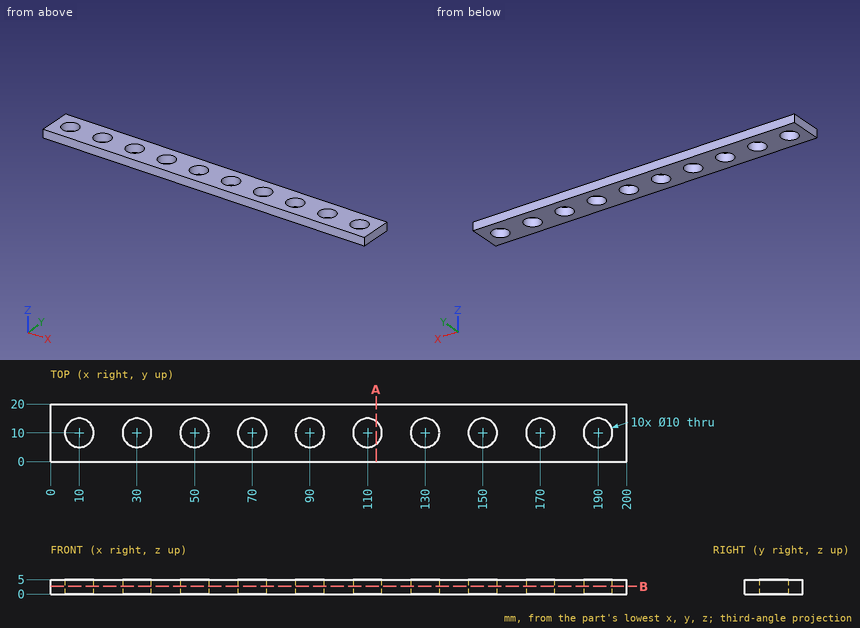
Geometry: see drawing. Coordinates: mm, zero at the bounding-box minimum. Round coordinates to 2 decimals unless told otherwise and drop trailing zeros. Write each loop counter-clockwise with the first axis right and the second up, starting at its lowest first coordinate (ties: lowest second). Pieces come first, ordered by that corner, then holes.
Item 1: Section query B-B (z = 2.65). Give the number of separate pieces and of enclosed holes in the cut face, plus the area to 3 significant figures.
Item 2: Material intervals for L1, parallel to Y at x = 190, z = 3.6; L2, parallel to Y at x = 148, z = 4.5, sorted ascending.
Item 3: Section query A-A (x = 113). Return loops of the section in (y, z), plus the area to 3 significant figures.
Completed:
1. separate pieces: 1
1. enclosed holes: 10
1. area: 3,210 mm2
2. L1: y = 0 to 5, 15 to 20
2. L2: y = 0 to 5.42, 14.58 to 20
3. outline: (0, 0) - (6, 0) - (6, 5) - (0, 5) - close; (14, 0) - (20, 0) - (20, 5) - (14, 5) - close
3. area: 60.0 mm2
